from build123d import *

# Parameters (mm, degrees)
SKETCH1_R           = 11.5
BOSS_EXTRUDE1_DEPTH = 5.5
SKETCH2_R           = 1
BOSS_EXTRUDE2_DEPTH = 3.25
FILLET1_R           = 0.5


with BuildPart() as part:
    # Sketch1 → Boss-Extrude1 (new, symmetric)
    with BuildSketch(Plane(origin=(0, 0, 0), x_dir=(1, 0, 0), z_dir=(0, 1, 0))):
        with Locations(Location((0, 0, 0), (0, 0, 270))):
            Circle(SKETCH1_R)
    extrude(amount=BOSS_EXTRUDE1_DEPTH, both=True)

    # Sketch2 → Boss-Extrude2 (add, symmetric)
    with BuildSketch(Plane.XZ.offset(5.5)):
        with Locations(Location((0, 0, 0), (0, 0, 90))):
            Circle(SKETCH2_R)
    extrude(amount=BOSS_EXTRUDE2_DEPTH, both=True)

    # Fillet1
    fillet1_edges = [part.edges().sort_by_distance(p)[0] for p in [
        (0, -5.5, -11.5),
    ]]
    fillet(fillet1_edges, radius=FILLET1_R)


solid = part.part
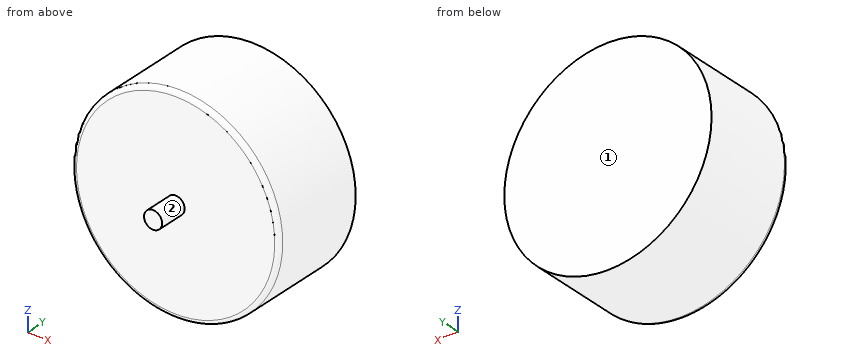
Design review of the part built by this model. Coordinates are the model's own, in mm. Face numbers are marked on the shaded views. A direction names the side the tool comes from. Give positions to 0.01 mm unless a question says otherwise; leave off trailing zeros. Write each loop counter-clockwise with the first axis right and the second up, starting at its lowest first coordinate (ties: lowest second). Pieces come first, ordered by that corner, then holes. Notation, with made-up numbers: M 48.5,29 L 70.5,29 A29 ccw 70.5,60 Z; hole C -4,11 d11. An arc over 180 degrees is marked long. Return JSON: item names as keys, results as strings. Group by question number.
Item 1: Take a section at A-A (x = 0). Give the boundary of the cut face in (y, z), plus the area to 3 significant figures.
Item 2: Take a section at C-C (y = -2.75). Give the boundary of the cut face in (x, z).
Item 3: Clearance check with flat-ended pins moving along their axes: pin 1 Ø4 at (x, z) = (-5, 3) entering from -Y; pin 2 Ø1 at (x, y) = (5, -4.5) entering from -Z; pin 3 Ø3 at (x, y) = (7, -6) entering from +Z. State where each tip first meets the part, or that it passes through.
Item 4: Wall thickness on line 1 along Y through (x, z) = (9.5, 4.75); line 2 along Z through (x, y) = (8.5, -0.25); line 3 along Z through (x, y) = (-9.5, 4): over which ranges is each line inside the solid? List them lowest first.
Item 5: Take a section at B-B (z = 0). Give the boundary of the cut face in (x, y).
Item 6: Tool access review of the marked faces 1 and 2: name each direction out of +Z, -Z, +X, -X, +Y, -Y from which nothing blocks a thin tool from reaching the whole face with its end or side.
Return value:
{
 "1": {"outline": "M -8.75,-1 L -5.5,-1 L -5.5,-11 A0.5 ccw -5,-11.5 L 5.5,-11.5 L 5.5,11.5 L -5,11.5 A0.5 ccw -5.5,11 L -5.5,1 L -8.75,1 Z", "area": "259 mm2"},
 "2": {"outline": "C 0,0 d23"},
 "3": {"pin 1": "stops at y = -5.5", "pin 2": "stops at z = -10.58", "pin 3": "stops at z = 9.92"},
 "4": {"line 1": "y = -5.5 to 5.5", "line 2": "z = -7.75 to 7.75", "line 3": "z = -6.48 to 6.48"},
 "5": {"outline": "M -11.5,-5 A0.5 ccw -11,-5.5 L -1,-5.5 L -1,-8.75 L 1,-8.75 L 1,-5.5 L 11,-5.5 A0.5 ccw 11.5,-5 L 11.5,5.5 L -11.5,5.5 Z"},
 "6": {"face 1": "+Z, -Z, +X, -X, +Y", "face 2": "-Y"}
}
